```python
from build123d import *

# Parameters (mm, degrees)
SKETCH1_R           = 12.7
BOSS_EXTRUDE1_DEPTH = 40.9448
CUT_EXTRUDE1_START  = -11.43
CUT_EXTRUDE1_DEPTH  = 11.43
CUT_EXTRUDE2_DEPTH  = 11.43


with BuildPart() as part:
    # Sketch1 → Boss-Extrude1 (new body)
    with BuildSketch(Plane(origin=(0, 0, 0), x_dir=(1, 0, 0), z_dir=(0, 1, 0))):
        with Locations(Location((0, 0, 0), (0, 0, 270))):
            Circle(SKETCH1_R)
    extrude(amount=BOSS_EXTRUDE1_DEPTH)

    # Sketch2 → Cut-Extrude1 (cut)
    with BuildSketch(Plane(origin=(0, 40.9448, 0), x_dir=(1, 0, 0), z_dir=(0, 1, 0)).offset(CUT_EXTRUDE1_START)):
        with BuildLine():
            Line((7.62, 10.16), (7.62, -10.16))
            ThreePointArc((7.62, -10.16), (0, -12.7), (-7.62, -10.16))
            Line((-7.62, -10.16), (-7.62, 10.16))
            ThreePointArc((-7.62, 10.16), (0, 12.7), (7.62, 10.16))
        make_face()
    extrude(amount=CUT_EXTRUDE1_DEPTH, mode=Mode.SUBTRACT)

    # Sketch3 → Cut-Extrude2 (cut)
    with BuildSketch(Plane.XZ):
        with BuildLine():
            Line((-7.62, 10.16), (-7.62, -10.16))
            ThreePointArc((-7.62, -10.16), (0, -12.7), (7.62, -10.16))
            Line((7.62, -10.16), (7.62, 10.16))
            ThreePointArc((7.62, 10.16), (0, 12.7), (-7.62, 10.16))
        make_face()
    extrude(amount=-CUT_EXTRUDE2_DEPTH, mode=Mode.SUBTRACT)


solid = part.part
```
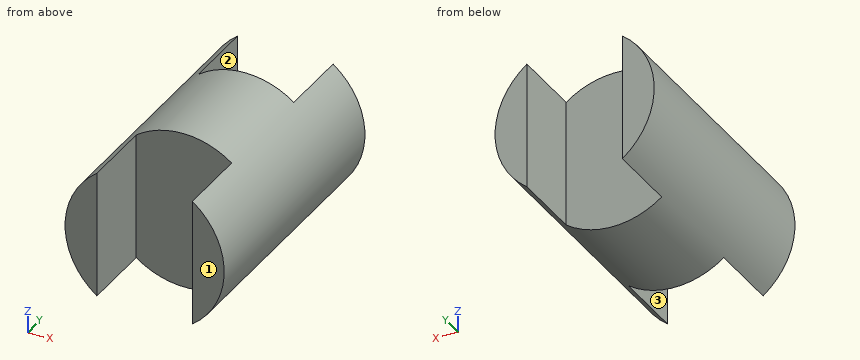
CAD build for the part. Positions are in the model's coordinates, mm. Face numbers are marked on the shaded views. A direction names the side the tool comes from. Coordinates: 2 decimals unless noted, no trailing zeros. Write each loop counter-clockwise with the first axis right and the second up, starting at its lowest first coordinate (ties: lowest second). Pieces come first, ordered by that corner, then holes.
(1) Drill centre lines: probe 1 along Y at (x, z) = (-1, 10.75); probe 2 along X at (y, z) = (7.5, 8.75); probe 3 along X at (y, z) = (37, -1.5). Where is each one in solid material? Low to high.
(2) Cut at B-B, the plane y = 5. List the corners of the cut face in (x, z), and give its area (3 significant figures).
(3) Cut at D-D, the plane y = 29. List the corners of the cut face in (x, z).
(4) 3-axis set-ups, long thin cutter, end or side, ignore diameter. For the marked faces 1, 2 and 3: which of +Z, -Z, +X, -X, +Y, -Y reach the whole face in a straight line?
(5) Flat gauge pins, fed straight in: pin 1 (1.5 mm diameter, centred on y = 10, z = -8, fed in from -X); pin 2 (3 mm diameter, centred on x = -3, z = -2, fed in from +Y); pin 3 (5.5 mm diameter, centred on y = 7.5, z = 3, fed in from -X). Where does each tip first touch, or does it go through?
(6) Cut at A-A, the plane z = 0. List the corners of the cut face in (x, y), and give its area (3 significant figures).
(7) Cut at C-C, the plane x = 0. List the corners of the cut face in (y, z).
Geometry says:
1. probe 1: y = 11.43 to 29.51
1. probe 2: x = -9.2 to -7.62, 7.62 to 9.2
1. probe 3: x = -12.61 to -7.62, 7.62 to 12.61
2. outline: (-7.62, -10.16) - (-7.62, 10.16) arc R12.7 ccw to start; (7.62, -10.16) arc R12.7 ccw to (7.62, 10.16) - close
2. area: 144 mm2
3. outline: circle Ø25.4 at (0, 0)
4. face 1: +Z, -Z, +X, -X, -Y
4. face 2: +Z, -Z, +Y
4. face 3: +Z, -Z, -Y
5. pin 1: stops at x = -10.43
5. pin 2: stops at y = 29.51
5. pin 3: stops at x = -12.7
6. outline: (-12.7, 0) - (-7.62, 0) - (-7.62, 11.43) - (7.62, 11.43) - (7.62, 0) - (12.7, 0) - (12.7, 40.94) - (7.62, 40.94) - (7.62, 29.51) - (-7.62, 29.51) - (-7.62, 40.94) - (-12.7, 40.94) - close
6. area: 692 mm2
7. outline: (11.43, -12.7) - (29.51, -12.7) - (29.51, 12.7) - (11.43, 12.7) - close
